Part model, mm, in its own coordinate system. Give positions to 0.01 mm unless a question says otherwise; leave off trailing zeros. Write each loop counter-clockwise with the first axis right and the second up, starting at its lowest first coordinate (ties: lowest second). Pieces come first, ordered by that corner, then holes.
```python
from build123d import *

# Parameters (mm, degrees)
SKETCH_1_R      = 47.5
SKETCH_1_R_2    = 44.5
EXTRUDE_2_DEPTH = 10
EXTRUDE_START   = -3
SKETCH_2_R      = 44.5
SKETCH_2_R_2    = 43.5
EXTRUDE_3_DEPTH = 3
FILLET_1_R      = 2
SKETCH_3_R      = 44.5
SKETCH_3_R_2    = 43.5
EXTRUDE_4_DEPTH = 3
FILLET_2_R      = 2


with BuildPart() as part:
    # 草图1 → 凸台-拉伸2 (new body)
    with BuildSketch(Plane.XY):
        Circle(SKETCH_1_R)
        Circle(SKETCH_1_R_2, mode=Mode.SUBTRACT)
    extrude(amount=EXTRUDE_2_DEPTH)

    # 草图2 → 凸台-拉伸3 (add)
    with BuildSketch(Plane.XY.offset(10).offset(EXTRUDE_START)):
        Circle(SKETCH_2_R)
        Circle(SKETCH_2_R_2, mode=Mode.SUBTRACT)
    extrude(amount=EXTRUDE_3_DEPTH)

    # 圆角1
    # the kernel refuses this fillet: 2 mm, written as the material it adds along each edge
    with BuildSketch(Plane(origin=(0, 0, 7), x_dir=(1, 0, 0), z_dir=(0, -1, 0))) as fillet_1_piece_1:
        with BuildLine():
            CenterArc((42.5, -1.732050808), FILLET_1_R, 0, 60)
            Line((43.5, 0), (43.52, 0.034641016))
            ThreePointArc((43.52, 0.034641016), (44, 0.04), (44.5, 0.04))
            Line((44.5, 0.04), (44.54, 0))
            Line((44.54, 0), (44.54, -1.732050808))
            Line((44.54, -1.732050808), (44.5, -1.732050808))
        make_face()
    revolve(axis=Axis((0, 0, 7), (0, 0, 1)))

    # 草图3 → 凸台-拉伸4 (add)
    with BuildSketch(Plane(origin=(0, 0, 0), x_dir=(-1, 0, 0), z_dir=(0, 0, -1))):
        Circle(SKETCH_3_R)
        with Locations(Location((0, 0, 0), (0, 0, 180))):
            Circle(SKETCH_3_R_2, mode=Mode.SUBTRACT)
    extrude(amount=-EXTRUDE_4_DEPTH)

    # 圆角2
    # the kernel refuses this fillet: 2 mm, written as the material it adds along each edge
    with BuildSketch(Plane(origin=(0, 0, 3), x_dir=(1, 0, 0), z_dir=(0, 1, 0))) as fillet_2_piece_1:
        with BuildLine():
            CenterArc((42.5, -1.732050808), FILLET_2_R, 0, 60)
            Line((43.5, 0), (43.52, 0.034641016))
            ThreePointArc((43.52, 0.034641016), (44, 0.04), (44.5, 0.04))
            Line((44.5, 0.04), (44.54, 0))
            Line((44.54, 0), (44.54, -1.732050808))
            Line((44.54, -1.732050808), (44.5, -1.732050808))
        make_face()
    revolve(axis=Axis((0, 0, 3), (0, 0, -1)))


solid = part.part
```
1) Pin check, flat tips, straight feed: pin 1 Ø3 at (y, z) = (-8, 1.5) entering from -X; pin 2 Ø2 at (x, z) = (36, 2) entering from +Y; pin 3 Ø5 at (y, z) = (-29, 6.5) entering from -X. Stop position of each tip, or through.
Answers follow:
pin 1: stops at x = -47.05
pin 2: stops at y = 32.11
pin 3: stops at x = -39.42
2) Two-plate mould, pull along X, no slides. Class faces 1 (the face through (-32.798, 30.075, 4.996)), 2 (the face through (-20.9, -38.5, 0)), 3 (the face through (-5.66, 43.13, 8.48)), 4 (the face through (-10.3, -46.37, 4.93)): +X half, -X half, draft (parallel to the pull), parting line (faces both ways), or undercut.
Answers follow:
face 1: undercut
face 2: draft
face 3: undercut
face 4: parting line
3) Saw through at C-C, the plane z = 1.5. Write the cut outline in (x, y), then the cut area to 3 significant figures.
Answers follow:
outline: circle Ø95 at (0, 0); hole circle Ø87 at (0, 0)
area: 1,140 mm2
4) Saw through at A-A, the plane x = 0. Write the cut outline in (y, z).
Answers follow:
outline: (-47.5, 0) - (-43.5, 0) - (-43.5, 3) arc R2 cw to (-44.5, 4.73) - (-44.5, 5.27) arc R2 cw to (-43.5, 7) - (-43.5, 10) - (-47.5, 10) - close; (43.5, 0) - (47.5, 0) - (47.5, 10) - (43.5, 10) - (43.5, 7) arc R2 cw to (44.5, 5.27) - (44.5, 4.73) arc R2 cw to (43.5, 3) - close
5) Wall check: L1, parallel to Y at x = 0, z = 5.15; L2, parallel to Y at x = 0, z = 9; L3, parallel to X at y = -38, z = 9.25. Give the ranges that are in metal, low to high.
Answers follow:
L1: y = -47.5 to -44.5, 44.5 to 47.5
L2: y = -47.5 to -43.5, 43.5 to 47.5
L3: x = -28.5 to -21.17, 21.17 to 28.5
